Work out the finished part from the listing and answer in its coordinate system (mm). A direction names the side the tool comes from. Give positions to 0.01 mm unless a question says otherwise; leave off trailing zeros. Loops run counter-clockwise (first coordinate to the right, second up) from the corner with the lowest first, then second, coordinate; pieces in that order, holes last. Notation, with made-up numbers: (74, -39.5) - (125, -39.5) arc R14 cw to (125, -30.5) - close; hole circle Ø2 at (51, 61.25). An arc over 180 degrees is marked (long way). Use CSV: the item, a comma, the result in double quotes.
from build123d import *

# Parameters (mm, degrees)
F0_W     = 177.8
F0_H     = 355.6
F2_DEPTH = 12.7
F1_W     = 147.32
F1_H     = 96.52
F4_DEPTH = 12.701
F8_W     = 152.4
F8_H     = 101.6
F9_DEPTH = 9.525


# Not quite as in the source:
# - a length typed as a fraction of an inch, garbled in the dataset ("3 / 203.2 mm" for 3/8 in), is restored


with BuildPart() as f2:
    # F0 (on Top) → F2 (new body)
    with BuildSketch(Plane.XY):
        Rectangle(F0_W, F0_H)
    extrude(amount=-F2_DEPTH)

    # F1 (on face) → F4 (cut, through all)
    with BuildSketch(Plane.XY):
        with Locations((0, -114.3)):
            Rectangle(F1_W, F1_H)
        Rectangle(F1_W, F1_H)
        with Locations((0, 114.3)):
            Rectangle(F1_W, F1_H)
    extrude(amount=-F4_DEPTH, mode=Mode.SUBTRACT)

    # F8 (on face) → F9 (cut)
    with BuildSketch(Plane(origin=(0, 0, -12.7), x_dir=(1, 0, 0), z_dir=(0, 0, -1))):
        with Locations((0, -114.3)):
            Rectangle(F8_W, F8_H)
        Rectangle(F8_W, F8_H)
        with Locations((0, 114.3)):
            Rectangle(F8_W, F8_H)
    extrude(amount=-F9_DEPTH, mode=Mode.SUBTRACT)


solid = f2.part
Item 1: For faces 1 (the flat face through (0, 54, -12.7)), 2 (the flat face through (-76.2, 1, -8)), determine the directions among +Z, -Z, +X, -X, +Y, -Y from which every point of the face is accessible in a straight line to the end or side of a thin tool.
Determined:
face 1,"-Z, +X, -X, +Y, -Y"
face 2,"-Z"
Item 2: A cutting plane is placed at B-B on y = 34. Determine the outline of the cut face in (x, z) (3 decimals).
Determined:
outline,"(-88.9, -12.7) - (-76.2, -12.7) - (-76.2, -3.175) - (-73.66, -3.175) - (-73.66, 0) - (-88.9, 0) - close; (73.66, -3.175) - (76.2, -3.175) - (76.2, -12.7) - (88.9, -12.7) - (88.9, 0) - (73.66, 0) - close"
Item 3: Find the intervals of material crossed by line 1 (Y direction, x = 33.5, z = -8.5); line 2 (Y direction, x = -30, z = -1.75); line 3 (X direction, y = -88, z = -10.5), in increasing order.
Determined:
line 1,"y = -177.8 to -165.1, -63.5 to -50.8, 50.8 to 63.5, 165.1 to 177.8"
line 2,"y = -177.8 to -162.56, -66.04 to -48.26, 48.26 to 66.04, 162.56 to 177.8"
line 3,"x = -88.9 to -76.2, 76.2 to 88.9"
Item 4: A cutting plane is placed at C-C on z = -10.25. Determine the outline of the cut face in (x, y), and give its area (3 significant figures).
Determined:
outline,"(-88.9, -177.8) - (88.9, -177.8) - (88.9, 177.8) - (-88.9, 177.8) - close; hole (-76.2, -165.1) - (76.2, -165.1) - (76.2, -63.5) - (-76.2, -63.5) - close; hole (-76.2, -50.8) - (76.2, -50.8) - (76.2, 50.8) - (-76.2, 50.8) - close; hole (-76.2, 63.5) - (76.2, 63.5) - (76.2, 165.1) - (-76.2, 165.1) - close"
area,"16,800 mm²"
Item 5: Given P1, Ø10, axis at x = 7.5, y = 40.5, coming from the +Z side; P2, Ø5, axis at x = 67, y = -57.5, coming from the +Z side, each flat-ended and moving along its own axis, determine where each tip first touches the part or whether it passes through.
Determined:
P1,"passes through"
P2,"stops at z = 0"
Item 6: The mould has two halves that part along X. Classify faces 3 (the flat face through (-1, 50.8, -8)), 4 (the flat face through (88.9, -2, -6)), 5 (the flat face through (-88.9, -2, -6)): pulls with the +X half, pulls with the -X half, needs draft (parallel to the pull), parting line crosses it, or undercut.
Determined:
face 3,"undercut"
face 4,"pulls with the +X half"
face 5,"pulls with the -X half"
Item 7: A cutting plane is placed at A-A on x = 10. Determine the outline of the cut face in (y, z) (3 decimals).
Determined:
outline,"(-177.8, -12.7) - (-165.1, -12.7) - (-165.1, -3.175) - (-162.56, -3.175) - (-162.56, 0) - (-177.8, 0) - close; (-66.04, -3.175) - (-63.5, -3.175) - (-63.5, -12.7) - (-50.8, -12.7) - (-50.8, -3.175) - (-48.26, -3.175) - (-48.26, 0) - (-66.04, 0) - close; (48.26, -3.175) - (50.8, -3.175) - (50.8, -12.7) - (63.5, -12.7) - (63.5, -3.175) - (66.04, -3.175) - (66.04, 0) - (48.26, 0) - close; (162.56, -3.175) - (165.1, -3.175) - (165.1, -12.7) - (177.8, -12.7) - (177.8, 0) - (162.56, 0) - close"
